Read the model definition and answer for the solid it produces. Units are mm, in the model's axes. A direction names the side the tool comes from. Give positions to 0.01 mm unless a question says otherwise; leave off trailing zeros. Loops run counter-clockwise (first coordinate to the right, second up) from the corner with the lowest first, then second, coordinate; pieces in that order, holes last. Notation, with made-up numbers: (-6.5, 46) -> (7.5, 46) arc R22 cw to (7.5, 82) -> close; hole circle Ø10 at (12.25, 6.5). An arc over 180 degrees is marked (long way). Return JSON: item names as keys, results as strings. Group by question number.
from build123d import *

# Parameters (mm, degrees)
CROQUIS6_R                 = 2.5
CORTAR_EXTRUIR1_DEPTH      = 26
CORTAR_EXTRUIR1_DEPTH_BACK = 26
CORTAR_EXTRUIR3_DEPTH      = 26.0000001
CORTAR_EXTRUIR3_DEPTH_BACK = 26.0000001


with BuildPart() as part:
    # Croquis3 → Revolución10 (revolve)
    with BuildSketch(Plane(origin=(0, 0, 0), x_dir=(1, 0, 0), z_dir=(0, 1, 0))):
        with BuildLine():
            Line((-38.081992127, 0), (161.918007873, 0))
            Line((161.918007873, 0), (161.918007873, 25))
            Line((161.918007873, 25), (-13.081992127, 25))
            ThreePointArc((-13.081992127, 25), (-30.759661656, 17.67766953), (-38.081992127, 0))
        make_face()
    revolve(axis=Axis((-38.081992127, 0, 0), (1, 0, 0)))

    # Croquis6 → Cortar-Extruir1 (cut, two sides)
    with BuildSketch(Plane.XY) as cortar_extruir1_sk:
        with Locations((156.918007873, 0)):
            Circle(CROQUIS6_R)
    extrude(amount=CORTAR_EXTRUIR1_DEPTH, mode=Mode.SUBTRACT)
    extrude(cortar_extruir1_sk.sketch, amount=-CORTAR_EXTRUIR1_DEPTH_BACK, mode=Mode.SUBTRACT)

    # Croquis9 → Cortar-Extruir3 (cut, two sides)
    with BuildSketch(Plane(origin=(0, 0, 0), x_dir=(1, 0, 0), z_dir=(0, 1, 0))) as cortar_extruir3_sk:
        with BuildLine():
            Line((161.918007873, 20), (161.918007873, -20))
            Line((161.918007873, -20), (151.918007873, -20))
            ThreePointArc((151.918007873, -20), (131.918007873, 0), (151.918007873, 20))
            Line((151.918007873, 20), (161.918007873, 20))
        make_face()
    extrude(amount=CORTAR_EXTRUIR3_DEPTH, mode=Mode.SUBTRACT)
    extrude(cortar_extruir3_sk.sketch, amount=-CORTAR_EXTRUIR3_DEPTH_BACK, mode=Mode.SUBTRACT)


solid = part.part
1. Section A-A on y = 0 is taken. Determine the outline of the cut face in (x, z), then the cut area to 3 significant figures.
2. Which of the six approach directions +Z, -Z, +X, -X, +Y, -Y give full straight-line access (tool end or side, diameter ignored) to faces 4 (the flat face through (154, 0, -20)), 5 (the cylindrical face through (154.934, -1.521, -22.465))?
3. Section D-D on y = 12 is taken. Determine the outline of the cut face in (x, z), then the cut area to 3 significant figures.
4. Section C-C on z = 0 is taken. Determine the outline of the cut face in (x, y), then the cut area to 3 significant figures.
5. Flat-ended cylindrical pins translate along their axes: pin 1 Ø10 at (x, y) = (23.5, -17.5) entering from -Z; pin 2 Ø1.5 at (x, z) = (84, 4.5) entering from -Y; pin 3 Ø1.5 at (y, z) = (6.5, 2.5) entering from -X; pin 4 Ø11 at (x, y) = (155.5, 3) entering from -Z. Find the tip coordinate at first contact, or state that the pin passes through.
6. Section B-B on x = 139 is taken. Determine the outline of the cut face in (y, z).
7. Determine the mould class of faces 1 (the flat face through (161.918, 0, 22)), 2 (the cylindrical face through (73.193, 7.509, -23.846)), 3 (the flat face through (154, 0, 20)) for opening direction Z: pulls with the +Z half, pulls with the -Z half, needs draft (parallel to the pull), parting line crosses it, or undercut.
8. Straight lines are drawn through the part: line 1 (X direction, y = 0, z = 23); line 2 (Z direction, x = 152.5, y = 13); line 3 (Z direction, x = 92.5, y = -20). For each, find the intervals that lie inside material, in ascending order. Write a range as from..to.
Completed:
{
 "1": {"outline": "(-13.08, -25) -> (154.42, -25) -> (154.42, -20) -> (151.92, -20) arc R20 cw to (151.92, 20) -> (154.42, 20) -> (154.42, 25) -> (-13.08, 25) arc R25 ccw to start; (159.42, -25) -> (161.92, -25) -> (161.92, -20) -> (159.42, -20) -> close; (159.42, 20) -> (161.92, 20) -> (161.92, 25) -> (159.42, 25) -> close", "area": "8,650 mm²"},
 "2": {"face 4": "+X, +Y, -Y", "face 5": "+Z, -Z"},
 "3": {"outline": "(-13.08, -21.93) -> (161.92, -21.93) -> (161.92, -20) -> (151.92, -20) arc R20 cw to (151.92, 20) -> (161.92, 20) -> (161.92, 21.93) -> (-13.08, 21.93) arc R21.93 ccw to start", "area": "7,400 mm²"},
 "4": {"outline": "(-13.08, -25) -> (131.92, -25) -> (131.92, 25) -> (-13.08, 25) arc R25 ccw to start", "area": "8,230 mm²"},
 "5": {"pin 1": "stops at z = -21.65", "pin 2": "stops at y = -24.72", "pin 3": "stops at x = -37.3", "pin 4": "stops at z = -25"},
 "6": {"outline": "(-19.8, -15.27) arc R25 ccw to (19.8, -15.27) -> close; (-19.8, 15.27) -> (19.8, 15.27) arc R25 ccw to start"},
 "7": {"face 1": "needs draft", "face 2": "parting line crosses it", "face 3": "undercut"},
 "8": {"line 1": "x = -22.88..154.42, 159.42..161.92", "line 2": "z = -21.35..-20, 20..21.35", "line 3": "z = -15..15"}
}
